Here's how the part is built. I have some questions about the finished solid (model axes, mm). Face numbers are marked on the shaded views. Round coordinates to 2 decimals unless told otherwise and drop trailing zeros. Write each loop counter-clockwise with the first axis right and the second up, starting at its lowest first coordinate (ties: lowest second). Pieces come first, ordered by that corner, then holes. Notation, with made-up numbers: (12.25, 78) -> (24.25, 78) arc R15 cw to (24.25, 83) -> close; hole circle Ø9 at (28.25, 16.5). An arc over 180 degrees is marked (long way). Put each result on its own line as item: value. Start each with the question number.
1. For pin 1 (3 mm diameter, centred on x = -5, y = -3.5, fed in from +Z); pin 2 (2 mm diameter, centred on x = -4, y = 5.5, fed in from +Z); pin 3 (5 mm diameter, centred on x = -3.5, z = 4, fed in from -Y), each with a flat end and sliding along its axis, tell me the tip position at first contact or that it passes through.
2. Suppose I cut it at A-A (x = 5.75). Please give me the cut outline in (y, z).
3. We'd pull the mould along Y, two halves only. Please class the marked faces 1 and 2: +Y half, -Y half, draft (parallel to the pull), parting line (faces both ways), or undercut.
4. I need wall thicknesses on probe 1 along Z at (x, y) = (4.25, 0); probe 2 along Z at (x, y) = (7.75, 2.75); probe 3 along X at (y, z) = (-3, 4.75). Which ranges of each line are inside material? Lowest first, please. Write a range as from..to.
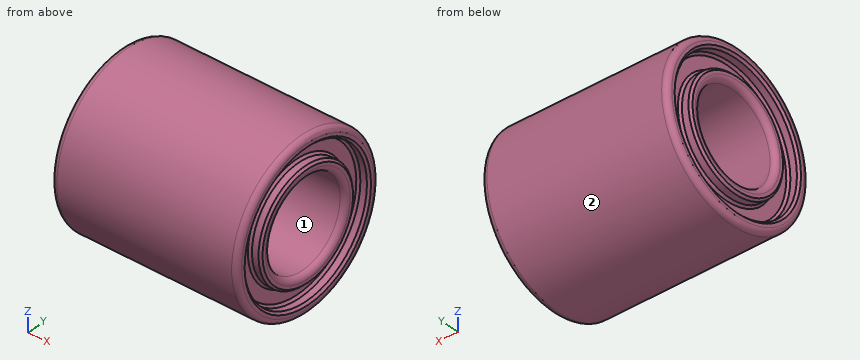
Autodesk Inventor part; units mm, degrees
ref_plane "YZ Plane" through (0, 0, 0) normal (1, 0, 0) x (0, 1, 0)
ref_plane "XZ Plane" through (0, 0, 0) normal (0, 1, 0) x (-1, 0, 0)
ref_plane "XY Plane" through (0, 0, 0) normal (0, 0, 1) x (1, 0, 0)
sketch "Эскиз1" plane through (0, 0, 0) normal (1, 0, 0) x (0, 1, 0)
  circle A0 centre (0, 0) radius 7.5
  circle A1 centre (0, 0) radius 4
  dimension "d0" = 15
  dimension "d1" = 8
extrude "Выдавливание1" add sketch "Эскиз1" along normal mid plane 17
sketch "Эскиз2" plane through (8.5, 0, 0) normal (1, 0, 0) x (0, 0, -1)
  circle A0 centre (0, 0) radius 5
  circle A1 centre (0, 0) radius 6.5
  dimension "d4" = 10
  dimension "d5" = 13
extrude "Выдавливание2" cut sketch "Эскиз2" against normal blind 1
sketch "Эскиз3" plane through (-8.5, 0, 0) normal (-1, 0, 0) x (0, 0, 1)
  circle A0 centre (0, 0) radius 6.5
  circle A1 centre (0, 0) radius 5
  dimension "d9" = 13
  dimension "d10" = 10
extrude "Выдавливание3" cut sketch "Эскиз3" against normal blind 1
fillet "Сопряжение1" radius 0.5 1 edges at (-8.5, -7.5, 0)
fillet "Сопряжение2" radius 0.5 3 edges at (-8.5, -4, 0) (8.5, -7.5, 0) (8.5, -4, 0)
chamfer "Фаска1" distance 0.2 angle 45 8 edges at (8.5, 0, 5) (8.5, 0, 6.5) (-8.5, 0, -5) (-8.5, 0, -6.5) (-7.5, 0, -5) (-7.5, 0, -6.5) (7.5, 0, 6.5) (7.5, 0, 5)
properties part number "LM8SUU"
Verdict:
1. pin 1: stops at z = 7.23
1. pin 2: stops at z = 6
1. pin 3: stops at y = -7.35
2. outline: circle Ø15 at (0, 0); hole circle Ø8 at (0, 0)
3. face 1: undercut
3. face 2: parting line
4. probe 1: z = -7.5..-4, 4..7.5
4. probe 2: z = -6.98..-5.89, -4.18..-2.9, 2.9..4.18, 5.89..6.98
4. probe 3: x = -7.5..7.5
